Input: part model. Units: mm. Frame: model coordinates. Face numbers are marked on the shaded views. A direction names the side the tool comes from. Round coordinates to 2 decimals unless told otherwise and drop trailing zeros. Loops run counter-clockwise (first coordinate to the right, second up) from the corner with the lowest first, then second, coordinate; pieces in that order, holes last. Notation, with made-up numbers: (-36, 46) -> (-12, 46) arc R7 cw to (-12, 53) -> close; hole circle Ø9 at (62.25, -16.75). An arc over 180 degrees is marked (long way). Answer as a JSON object with one key per item and string values.
```python
from build123d import *

# Parameters (mm, degrees)
F0_R      = 14.2875
F1_DEPTH  = 5.08
F3_DEPTH  = 5.08
F4_COUNT  = 10
F5_R      = 9.525
F6_DEPTH  = 5.081
F7_DEPTH  = 5.081
F9_DEPTH  = 5.08
F10_COUNT = 3
F11_R     = 3.302
F12_DEPTH = 5.081


with BuildPart() as f1:
    # F0 (on Top) → F1 (new body)
    with BuildSketch(Plane.XY):
        Circle(F0_R)
    extrude(amount=F1_DEPTH)

    # F4: F3 ×10 about axis
    f4_axis = Axis((0, 0, 5.08), (0, 0, 1))


with BuildPart() as f3:
    # F2 (on face) → F3 (new body, through all)
    with BuildSketch(Plane.XY.offset(5.08)):
        with BuildLine():
            Line((-4.393811939, 13.5947116911), (-0.0222334703, 14.2871017002))
            ThreePointArc((-0.0222334703, 14.2871017002), (0.0536070974, 18.934616917), (-3.4776602758, 21.957082834))
            ThreePointArc((-3.4776602758, 21.957082834), (-5.9021017886, 17.9913252983), (-4.393811939, 13.5947116911))
        make_face()
    extrude(amount=-F3_DEPTH)


with BuildPart() as f1_1:
    add(f1.part)
    for i in range(1, F4_COUNT):
        add(f3.part.rotate(f4_axis, i * 360 / F4_COUNT))

    # F5 (on face) → F6 (cut, through all)
    with BuildSketch(Plane.XY.offset(5.08)):
        Circle(F5_R)
    extrude(amount=-F6_DEPTH, mode=Mode.SUBTRACT)

    # F5 (on face) → F7 (cut, through all)
    with BuildSketch(Plane.XY.offset(5.08)):
        Circle(F5_R)
    extrude(amount=-F7_DEPTH, mode=Mode.SUBTRACT)



with BuildPart() as f9:
    # F8 (on face) → F9 (new body, through all)
    with BuildSketch(Plane.XY.offset(5.08)):
        with BuildLine():
            Line((-1.6539988923, 9.3802938474), (-1.1026659282, 6.2535292316))
            ThreePointArc((-1.1026659282, 6.2535292316), (0, -6.35), (1.1026659282, 6.2535292316))
            Line((1.1026659282, 6.2535292316), (1.6539988923, 9.3802938474))
            ThreePointArc((1.6539988923, 9.3802938474), (0, 9.525), (-1.6539988923, 9.3802938474))
        make_face()
    extrude(amount=-F9_DEPTH)


with BuildPart() as f1_2:
    add(f1_1.part)

    add(f3.part)  # F10 merges F3

    add(f9.part)  # F10 merges F9
    # F10: F9 ×3 about axis
    f10_axis = Axis((0, 0, 5.08), (0, 0, 1))
    for i in range(1, F10_COUNT):
        add(f9.part.rotate(f10_axis, i * 360 / F10_COUNT))

    # F11 (on face) → F12 (cut, through all)
    with BuildSketch(Plane.XY.offset(5.08)):
        Circle(F11_R)
    extrude(amount=-F12_DEPTH, mode=Mode.SUBTRACT)


solid = f1_2.part
```
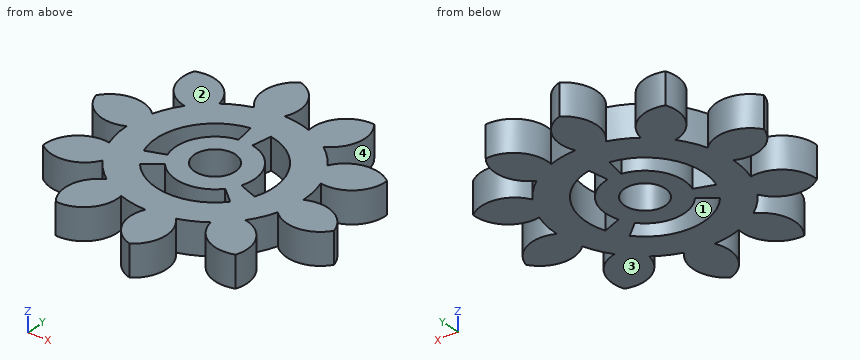
1) Reachability of the marked faces 1 and 2 from +Z, -Z, +X, -X, +Y, -Y: full face, straight path, thin tool, end or side. Return the list, or none.
Output:
{"face 1": "+Z, -Z", "face 2": "+Z, +X, -X, +Y, -Y"}
2) Section A-A, the plane y = 19. Output: boundary loops of the cut face in (x, z), plus the area to 3 significant figures.
Output:
{"outline": "(-5.69, 0) -> (0.02, 0) -> (0.02, 5.08) -> (-5.69, 5.08) -> close; (6.97, 0) -> (10.63, 0) -> (10.63, 5.08) -> (6.97, 5.08) -> close", "area": "47.6 mm^2"}
3) Draft query along Y for the marked faces 3 and 4. Return one class per face: +Y half, -Y half, draft (parallel to the pull), parting line (faces both ways), or undercut.
Output:
{"face 3": "draft", "face 4": "undercut"}
4) Section D-D, the plane z = 1.6. Count the separate pieces of the cut face and the enclosed holes in it, plus the area to 3 significant figures.
Output:
{"separate pieces": "1", "enclosed holes": "4", "area": "881 mm^2"}
5) Section C-C, the plane y = 2. Output: boundary loops of the cut face in (x, z).
Output:
{"outline": "(-21.3, 0) -> (-9.31, 0) -> (-9.31, 5.08) -> (-21.3, 5.08) -> close; (-6.03, 0) -> (-2.63, 0) -> (-2.63, 5.08) -> (-6.03, 5.08) -> close; (2.63, 0) -> (6.03, 0) -> (6.03, 5.08) -> (2.63, 5.08) -> close; (9.31, 0) -> (14.15, 0) -> (14.15, 5.08) -> (9.31, 5.08) -> close"}
6) Contact query for flat-ended pins moving along their axis: P1, Ø1.5, axis at y = 0.5, z = 4.5, coming from the -X side; P2, Ø6, axis at x = -15.5, y = -17.5, coming from the -Z side; P3, Ø3, axis at y = -15, z = 2, coming from the +X side; P4, Ø3, axis at x = 4.5, z = 3.5, coming from the +Y side. Output: stop coordinate, or through.
Output:
{"P1": "stops at x = -20.73", "P2": "passes through", "P3": "stops at x = 16.07", "P4": "stops at y = 18.23"}
7) Ray query, probe 1 along X at (y, z) = (2, 2.6); probe 2 along X at (y, z) = (4, 1.1); probe 3 along X at (y, z) = (-2, 4.1). Return the intervals inside material, ascending.
Output:
{"probe 1": "x = -21.3 to -9.31, -6.03 to -2.63, 2.63 to 6.03, 9.31 to 14.15", "probe 2": "x = -21.57 to -8.64, -4.93 to 4.93, 8.64 to 13.72", "probe 3": "x = -14.15 to -9.31, -6.03 to -2.63, 2.63 to 6.03, 9.31 to 21.3"}
8) Section B-B, the plane x = -18. Output: boundary loops of the cut face in (y, z).
Output:
{"outline": "(-11.05, 0) -> (-5.78, 0) -> (-5.78, 5.08) -> (-11.05, 5.08) -> close; (-0.38, 0) -> (5.9, 0) -> (5.9, 5.08) -> (-0.38, 5.08) -> close"}
